```python
from build123d import *

# Parameters (mm, degrees)
F2_R    = 1
F3_SIZE = 0.5


with BuildPart() as f1:
    # F0 (on Front) → F1 (revolve)
    with BuildSketch(Plane.XZ):
        Polygon((-5, -10), (0, -10), (0, 6.47346), (-20, 10), (-20, 45), (-25, 45), (-25, 0), (-5, 0), align=None)
    revolve(axis=Axis((0, 0, -1.76327), (0, 0, -1)))

    # F2
    f2_edges = [f1.edges().sort_by_distance(p)[0] for p in [
        (5, 0, 0),
    ]]
    fillet(f2_edges, radius=F2_R)

    # F3
    f3_edges = [f1.edges().sort_by_distance(p)[0] for p in [
        (5, 0, -10),
        (25, 0, 0),
        (25, 0, 45),
        (20, 0, 45),
    ]]
    chamfer(f3_edges, length=F3_SIZE)


solid = f1.part
```
Could you check a few things on this model? Use its own coordinates, in mm. A direction names the side the tool comes from. Round coordinates to 2 decimals unless told otherwise and drop trailing zeros. Loops run counter-clockwise (first coordinate to the right, second up) from the corner with the lowest first, then second, coordinate; pieces in that order, holes last. Notation, with made-up numbers: (89, 38) - (108, 38) arc R20 cw to (108, 66) - close; hole circle Ø9 at (-36, -5.75). An arc over 180 degrees is marked (long way). Answer in a Markdown table with one row per item. Add a question column.
(1) For faces 1 (the face through (-5, -5, 0)), 2 (the face through (-6, -20, 45)), which set-ups out of +Z, -Z, +X, -X, +Y, -Y let a thin tool reach every point of the face, with its end or its side?
(2) If we mould it in two halves opening along X, with no side actions, what happens to faces 3 (the face through (0, 0, -10)), 4 (the face through (1.08, -4.88, -5.31)), 5 (the face through (4.336, -19.524, 27.492))? For each: pulls with the +X half, pulls with the -X half, needs draft (parallel to the pull), parting line crosses it, or undercut.
(3) If we section it at C-C (z = 2.5): Please give me the cut outline in (x, y).
(4) I'm going to push flat-ended pins straight in: pin 1 (6 mm diameter, centred on y = -20, z = 30, fed in from -X); pin 2 (3 mm diameter, centred on y = -5, z = -2.5, fed in from -X); pin 3 (4 mm diameter, centred on y = 1.5, z = 24.5, fed in from +X); pin 4 (8 mm diameter, centred on y = 7, z = 1, fed in from -X). Where does each tip first touch, or does it pass through?
(5) If we section it at A-A (z = 26): Please give me the cut outline in (x, y), plus the area to 3 significant figures.
(6) If we section it at B-B (z = -3.5): Please give me the cut outline in (x, y), plus the area to 3 significant figures.
(7) I need wall thicknesses on line 1 along Y through (x, z) = (0, 33.5); line 2 along Z through (x, y) = (-16, 18); line 3 along X through (y, z) = (-3.5, 40.5). Which ranges of each line are inside material? Lowest first, please.
Model answer:
| question | item | result |
|---|---|---|
| 1 | face 1 | -Z |
| 1 | face 2 | +Z, +X, -X, +Y, -Y |
| 2 | face 3 | needs draft |
| 2 | face 4 | parting line crosses it |
| 2 | face 5 | undercut |
| 3 | outline | circle Ø50 at (0, 0) |
| 4 | pin 1 | stops at x = -18.33 |
| 4 | pin 2 | stops at x = -3.57 |
| 4 | pin 3 | stops at x = 25 |
| 4 | pin 4 | stops at x = -24.82 |
| 5 | outline | circle Ø50 at (0, 0); hole circle Ø40 at (0, 0) |
| 5 | area | 707 mm² |
| 6 | outline | circle Ø10 at (0, 0) |
| 6 | area | 78.5 mm² |
| 7 | line 1 | y = -25 to -20, 20 to 25 |
| 7 | line 2 | z = 0 to 45 |
| 7 | line 3 | x = -24.75 to -19.69, 19.69 to 24.75 |
